Build history of the part. All positions in model axes, mm. A direction names the side the tool comes from. Coordinates: 2 decimals unless noted, no trailing zeros. Write each loop counter-clockwise with the first axis right and the second up, starting at its lowest first coordinate (ties: lowest second). Pieces come first, ordered by that corner, then holes. Notation, with made-up numbers: (51.5, -31.5) -> (60.5, -31.5) arc R19 ccw to (60.5, -11.5) -> close; hole circle Ø7 at (-14.75, 86.5). An arc over 180 degrees is marked (long way). Write each question's results on one line, items separated by ' | '. Start each with the question number.
Q1. Saw through at D-D on x = 0. Give the cut face in (y, z), and give its area (3 significant figures).
Q2. Drill centre lines: line 1 (Y direction, x = 10.2, z = 12.55); line 2 (Z direction, x = -5.75, y = 7); line 3 (X direction, y = 6.5, z = 11). Where is each one in solid material? Low to high.
Q3. Saw through at A-A on x = -10.2. Give the cut face in (y, z).
Q4. Tool access for faces 4 (the face through (0, -6.25, 13)), 5 (the face through (7.6, -7.25, 4.6)), 6 (the face through (1.124, 11, 6)), 7 (the face through (0, 0, 0)), 8 (the face through (-7.6, -7.25, 5.1)): list every direction of +Z, -Z, +X, -X, +Y, -Y with a clear straight run to the whole face (end or side of a thin tool).
Q5. Two-plate mould, pull along X, no slides. Class faces 1 (the face through (-5.5, -12.7, 0.9)), 2 (the face through (7.75, 0, 6)), 3 (the face through (10.677, 2.9, 13.014)): released by +X, released by -X, zero draft, split by the parting line, or undercut.
Q6. Drop flat-ended pins along their axis: pin 1 Ø2 at (y, z) = (9, 6) entering from +X; pin 2 Ø3 at (y, z) = (-2.5, 4) entering from -X; pin 3 Ø5 at (y, z) = (8.5, 1.5) entering from +X. Give the stop position or say it passes through.
Q7. Saw through at C-C on z = 6. Give the cut face in (x, y).
Q8. Saw through at B-B on y = 6.75. Give the cut face in (x, z).
Autodesk Inventor part; units mm, degrees
ref_plane "YZ Plane" through (0, 0, 0) normal (1, 0, 0) x (0, 1, 0)
ref_plane "XZ Plane" through (0, 0, 0) normal (0, 1, 0) x (-1, 0, 0)
ref_plane "XY Plane" through (0, 0, 0) normal (0, 0, 1) x (1, 0, 0)
sketch "Skizze1" plane through (0, 0, 0) normal (0, 0, 1) x (1, 0, 0)
  line L0 (7.75, -7.25) -> (-7.75, -7.25)
  line L1 (-7.75, -7.25) -> (-7.75, 7.25)
  line L2 (-7.75, 7.25) -> (7.75, 7.25)
  line L3 (7.75, 7.25) -> (7.75, -7.25)
  line L4 (7.75, -7.25) -> (-7.75, 7.25) construction
  line L5 (-7.75, -7.25) -> (7.75, 7.25) construction
  point P0 (0, 0)
  dimension "d0" = 15.5
  dimension "d1" = 14.5
extrude "Extrusion1" add sketch "Skizze1" along normal blind 12
sketch "Skizze2" plane through (0, 0, 12) normal (0, 0, 1) x (1, 0, 0)
  line L0 (12, -6.25) -> (-12, -6.25)
  line L1 (-12, -6.25) -> (-12, 9.75)
  line L2 (-12, 9.75) -> (12, 9.75)
  line L3 (12, 9.75) -> (12, -6.25)
  line L4 (12, -6.25) -> (-12, 9.75) construction
  line L5 (-12, -6.25) -> (12, 9.75) construction
  line L6 (7.75, 7.25) -> (-7.75, 7.25)
  point P0 (0, 0)
  point P1 (0, 1.75)
  dimension "d4" = 24
  dimension "d5" = 16
  dimension "d6" = 2.5
extrude "Extrusion2" add sketch "Skizze2" along normal blind 2
sketch "Skizze3" plane through (-7.75, 7.25, 0) normal (0, 1, 0) x (1, 0, 0)
  line L0 (15.5, 0) -> (0, 0)
  line L1 (0, 0) -> (0, -12)
  line L2 (15.5, -12) -> (0, -12)
  line L3 (15.5, 0) -> (15.5, -12)
  circle A0 centre (7.75, -6) radius 1.5
  line L4 (8.8745, -5.0073) -> (8.8745, -6.9927)
  point P0 (7.75, 0)
  dimension "d9" = 3
  dimension "d10" = 1.1245
extrude "Extrusion3" add sketch "Skizze3" along normal blind 7 contours L4 A0 picked at (7.9997, -6)
sketch "Skizze4" plane through (-7.75, -7.25, 0) normal (0, -1, 0) x (1, 0, 0)
  line L0 (0, 0) -> (15.5, 0)
  line L1 (15.5, 0) -> (15.5, 12)
  line L2 (0, 12) -> (15.5, 12)
  line L3 (0, 0) -> (0, 12)
  arc A0 (8.8745, 6.9927) -> (8.8745, 5.0073) centre (7.75, 6) ccw
  circle A1 centre (7.75, 6) radius 7.5
  point P0 (7.75, 0)
  dimension "d13" = 15
extrude "Extrusion4" add sketch "Skizze4" along normal blind 11 contours A1 L2 L0 | L0 A1 | A1 L2
sketch "Skizze5" plane through (0, 0, 14) normal (0, 0, 1) x (1, 0, 0)
  line L0 (12, 9.75) -> (-12, 9.75)
  line L1 (-12, 9.75) -> (-12, -6.25)
  line L2 (-12, -6.25) -> (12, -6.25)
  line L3 (12, -6.25) -> (12, 9.75)
  line L4 (-7.75, 7.25) -> (-7.75, -6.25)
  line L5 (7.75, -6.25) -> (7.75, 7.25)
  circle A0 centre (-10.2, -1.25) radius 0.5
  circle A1 centre (-10.2, 2.75) radius 0.5
  circle A2 centre (-10.2, 6.75) radius 0.5
  line L6 (0, 9.75) -> (0, -6.25)
  line L7 (12, 9.75) -> (12, -6.25)
  line L8 (7.75, 7.25) -> (7.75, -6.25)
  circle A3 centre (10.2, -1.25) radius 0.5
  circle A4 centre (10.2, 2.75) radius 0.5
  circle A5 centre (10.2, 6.75) radius 0.5
  point P0 (0, 0)
  dimension "d16" = 1
  dimension "d17" = 1
  dimension "d18" = 1
  dimension "d19" = 5
  dimension "d20" = 4
  dimension "d21" = 4
  dimension "d22" = 1.8
  dimension "d23" = 1.8
  dimension "d24" = 1.8
extrude "Extrusion5" cut sketch "Skizze5" against normal blind 11 contours A0 | A1 | A2 | A3 | A4 | A5
properties part number "00_Micro_Stepper_15mm_Gearbox"
Returned:
1) outline: (-18.25, -1.5) -> (-7.25, -1.5) -> (-7.25, 0) -> (7.25, 0) -> (7.25, 4.5) -> (14.25, 4.5) -> (14.25, 7.5) -> (7.25, 7.5) -> (7.25, 12) -> (9.75, 12) -> (9.75, 14) -> (-6.25, 14) -> (-6.25, 12) -> (-7.25, 12) -> (-7.25, 13.5) -> (-18.25, 13.5) -> close | area: 392 mm2
2) line 1: y = -6.25 to -1.75, -0.75 to 2.25, 3.25 to 6.25, 7.25 to 9.75 | line 2: z = 0 to 14 | line 3: x = -7.75 to 7.75
3) outline: (-6.25, 12) -> (-1.75, 12) -> (-1.75, 14) -> (-6.25, 14) -> close; (-0.75, 12) -> (2.25, 12) -> (2.25, 14) -> (-0.75, 14) -> close; (3.25, 12) -> (6.25, 12) -> (6.25, 14) -> (3.25, 14) -> close; (7.25, 12) -> (9.75, 12) -> (9.75, 14) -> (7.25, 14) -> close
4) face 4: +Z, +X, -X | face 5: +X, -Y | face 6: -Z, +X, +Y | face 7: -Z, +X, -X, +Y | face 8: -X, -Y
5) face 1: split by the parting line | face 2: released by +X | face 3: undercut
6) pin 1: stops at x = 1.12 | pin 2: stops at x = -7.75 | pin 3: stops at x = 7.75
7) outline: (-7.75, -7.25) -> (-7.5, -7.25) -> (-7.5, -18.25) -> (7.5, -18.25) -> (7.5, -7.25) -> (7.75, -7.25) -> (7.75, 7.25) -> (1.12, 7.25) -> (1.12, 14.25) -> (-1.5, 14.25) -> (-1.5, 7.25) -> (-7.75, 7.25) -> close
8) outline: (-12, 12) -> (-10.7, 12) -> (-10.7, 14) -> (-12, 14) -> close; (-9.7, 12) -> (-7.75, 12) -> (-7.75, 0) -> (7.75, 0) -> (7.75, 12) -> (9.7, 12) -> (9.7, 14) -> (-9.7, 14) -> close; (10.7, 12) -> (12, 12) -> (12, 14) -> (10.7, 14) -> close
